Input: part model. Units: mm. Frame: model coordinates. Coordinates: 2 decimals unless noted, no trailing zeros. Order: outer loops, then holes, each group sorted by start corner. A loop starts at its lowest first (then second) coordinate and runs counter-clockwise, first axis right, second up. Notation, with made-up numbers: M -27,23 L -8,23 A29 cw -8,57 Z; hole C -19,12.25 d4. An arc over 180 degrees is marked long. One line per item, written item: value.
```python
from build123d import *

# Parameters (mm, degrees)
F1_DEPTH    = 11.62886
F2_T1_DEPTH = 111.62886
F4_ANGLE    = -90


# Not quite as in the source:
# - a fillet or chamfer that OpenCascade refuses, or shapes differently, is made with other operations: its cross-section is extruded or revolved along the edge and cut away or added


with BuildPart() as f1:
    # F0 (on Top) → F1 (new body)
    with BuildSketch(Plane.XY):
        Polygon((45.4364679754, 42.3810482025), (0, 0), (98.7063497305, 0), (98.7063497305, 42.3810482025), align=None)
    extrude(amount=F1_DEPTH)

    # F2: fillet of radius 20 on 1 edges, made by hand

    # F2_s2 → F2_t1 (cut)
    with BuildSketch(Plane.XY.offset(-50)):
        with BuildLine():
            add(Edge.make_bspline(
                [(78.7063497305, 0), (98.7063497305, 0), (98.7063497305, 20)],
                knots=[0, 0, 0, 1, 1, 1], degree=2, weights=[1, 1, 1]))
            Line((98.7063497305, 20), (98.7063497305, 0))
            Line((98.7063497305, 0), (78.7063497305, 0))
        make_face()
    extrude(amount=F2_T1_DEPTH, mode=Mode.SUBTRACT)

    # F3: F1 across plane


with BuildPart() as f1_1:
    add(f1.part)
    add(f1.part.mirror(Plane.XZ))


with BuildPart() as f1_2:
    # F4: moved
    add(f1_1.part.rotate(Axis((22.7182339877, -21.1905241013, 11.62886), (-0.7312665459, 0.6820918111, 0)), F4_ANGLE))


solid = f1_2.part
```
(1) Cut plane D-D on y = -64. Output: boundary loops of the cut face in (x, z).
Data:
outline: M 68.61,41.19 L 78.54,47.96 L 68.61,55.75 Z
(2) Cut plane B-B on x = 35. Output: boundary loops of the cut face in (y, z).
Data:
outline: M -32.65,11.63 L -16.74,11.63 L -16.74,104.11 L -25.92,109.95 L -32.65,105.03 Z
(3) Cut plane A-A on y = -28. Output: boundary loops of the cut face in (x, z), plus the area to 3 significant figures.
Data:
outline: M 30.02,11.63 L 47.07,11.63 L 47.07,98.96 L 33.06,109.95 L 30.02,107.87 Z
area: 1,600 mm2
(4) Cut plane C-C on z = 33. Output: boundary loops of the cut face in (x, y), plus the area to 3 significant figures.
Data:
outline: M 1.09,-1.02 L 62.19,-58.01 L 70.12,-49.51 L 9.02,7.49 Z
area: 972 mm2
(5) First-contact query: pin 1 (3 mm diameter, centred on x = 16, y = -19.5, fed in from +Z); pin 2 (8 mm diameter, centred on x = 65, y = -45, fed in from +Z); pin 3 (10 mm diameter, centred on y = -19.5, z = 91, fed in from +X); pin 4 (1 mm diameter, centred on y = -7, z = 35.5, fed in from -X). Flat tips, straight axial feed; report the tip coordinate or a pass-through.
Data:
pin 1: passes through
pin 2: stops at z = 71.62
pin 3: stops at x = 43.32
pin 4: stops at x = 6.97
(6) Ray query, line 1 (Y direction, x = 48, z = 36.5); line 2 (Y direction, x = 57, z = 31.5); line 3 (X direction, y = -1, z = 38.5). Return the intervals inside material, ascending. Write a range as from..to.
Data:
line 1: y = -44.77..-28.87
line 2: y = -53.17..-37.26
line 3: x = 1.63..18.12
